```python
from build123d import *

# Parameters (mm, degrees)
SM_BASE_FLANGE_1_DEPTH = 80
CUT_EXTRUDE_1_DEPTH    = 35
FILLET_1_R             = 1
EXTRUDE_START          = -1.5
EXTRUDE_1_OUTLINE_R    = 4.25
EXTRUDE_1_DEPTH        = 1.5


# Read off the part's stored shape, not the designer's step: Бобышка-Вытянуть1
# Sheet-metal steps are written as plain solids
with BuildPart() as part:
    # Sketch 1 → Базовая кромка1 (new body)
    with BuildSketch(Plane(origin=(0, 0, 0), x_dir=(0, 0, -1), z_dir=(1, 0, 0))):
        with BuildLine():
            Line((-6, 25.5), (-6, 1))
            ThreePointArc((-6, 1), (-5.707106781, 0.292893219), (-5, 0))
            Line((-5, 0), (5, 0))
            ThreePointArc((5, 0), (5.707106781, 0.292893219), (6, 1))
            Line((6, 1), (6, 25.5))
            Line((6, 25.5), (7.5, 25.5))
            Line((7.5, 25.5), (7.5, 1))
            ThreePointArc((7.5, 1), (6.767766953, -0.767766953), (5, -1.5))
            Line((5, -1.5), (-5, -1.5))
            ThreePointArc((-5, -1.5), (-6.767766953, -0.767766953), (-7.5, 1))
            Line((-7.5, 1), (-7.5, 25.5))
            Line((-7.5, 25.5), (-6, 25.5))
        make_face()
    extrude(amount=SM_BASE_FLANGE_1_DEPTH)

    # Эскиз6 → Вырез-Вытянуть1 (cut)
    with BuildSketch(Plane.XY.offset(7.5)):
        Polygon((80, 25.5), (75.076809621, 25.5), (80, 5.5), align=None)
        with BuildLine():
            ThreePointArc((13.923190379, 25.5), (23.568323275, 11.075714714), (40, 5.5))
            Line((40, 5.5), (40, 25.5))
            Line((40, 25.5), (13.923190379, 25.5))
        make_face()
        with BuildLine():
            Line((40, 25.5), (40, 5.5))
            ThreePointArc((40, 5.5), (56.431676725, 11.075714714), (66.076809621, 25.5))
            Line((66.076809621, 25.5), (40, 25.5))
        make_face()
        Polygon((0, 5.5), (4.923190379, 25.5), (0, 25.5), align=None)
    extrude(amount=-CUT_EXTRUDE_1_DEPTH, mode=Mode.SUBTRACT)

    # Скругление1
    fillet_1_edges = [part.edges().sort_by_distance(p)[0] for p in [
        (75.076809621, 25.5, -6.75),
        (75.076809621, 25.5, 6.75),
        (13.923190379, 25.5, -6.75),
        (66.076809621, 25.5, -6.75),
        (13.923190379, 25.5, 6.75),
        (66.076809621, 25.5, 6.75),
        (4.923190379, 25.5, -6.75),
        (4.923190379, 25.5, 6.75),
    ]]
    fillet(fillet_1_edges, radius=FILLET_1_R)

    # Бобышка-Вытянуть1 outline → Бобышка-Вытянуть1 (cut)
    with BuildSketch(Plane.XZ.offset(1.5).offset(EXTRUDE_START)):
        with Locations((71, 0)):
            Circle(EXTRUDE_1_OUTLINE_R)
        with Locations((9, 0)):
            Circle(EXTRUDE_1_OUTLINE_R)
    extrude(amount=EXTRUDE_1_DEPTH, mode=Mode.SUBTRACT)


solid = part.part
```
Work out the finished part from the listing and answer in its coordinate system (mm). A direction names the side the tool comes from. Give positions to 0.01 mm unless a question says otherwise; leave off trailing zeros. Loops run counter-clockwise (first coordinate to the right, second up) from the corner with the lowest first, then second, coordinate; pieces in that order, holes last. Notation, with made-up numbers: (16.25, 27.25) -> (59.25, 27.25) arc R3 ccw to (59.25, 32.25) -> close; hole circle Ø10 at (3.25, 39). An arc over 180 degrees is marked (long way). Write item = value, one per line. Start each with the question number.
(1) Find the intervals of material crossed by probe 1 along Z at (x, y) = (71.5, 15); probe 2 along Y at (x, z) = (73, 4.75); probe 3 along Z at (x, y) = (9, -0.8), in increasing order. Write a range as from..to.
(2) Find section C-C on z = 0. Give the vertices of the cut face in (x, y).
(3) Find section A-A on x = 71. Give the vertices of the cut face in (y, z), and give its area (3 significant figures).
(4) Which of the six approach directions +Z, -Z, +X, -X, +Y, -Y give full straight-line access (tool end or side, diameter ignored) to faces 4 (the flat face through (39, 5, -6)), 5 (the cylindrical face through (39.44, -0.748, -6.787))?
(5) Given pin 1 Ø5 at (y, z) = (15, -4) entering from -X; pin 2 Ø1.5 at (x, z) = (55.5, -1) entering from +Y; pin 3 Ø6 at (y, z) = (13, -5) entering from +X; pin 4 Ø12 at (x, y) = (49, 20.5) entering from -Z, each flat-ended and moving along its own axis, determine where each tip first touches the part or whether it passes through.
(6) Find section D-D on x = 41. Give the vertices of the cut face in (y, z).
(7) The mould has two halves that part along Z. Classify faces 1 (the flat face through (39, 5, 6)), 2 (the cylindrical face through (39.44, -0.787, 6.748)), 3 (the flat face through (2.335, 14.985, -6.74)): +Z half, -Z half, draft (parallel to the pull), parting line (faces both ways), or undercut.
(8) Find section B-B on y = 16.75. Give the vertices of the cut face in (x, z), and give its area (3 significant figures).
From the geometry:
q1.probe_1 = -7.5..-6, 6..7.5
q1.probe_2 = -1.5..0
q1.probe_3 = -6.73..-4.25, 4.25..6.73
q2.outline = (0, -1.5) -> (4.75, -1.5) -> (4.75, 0) -> (0, 0) -> close; (13.25, -1.5) -> (66.75, -1.5) -> (66.75, 0) -> (13.25, 0) -> close; (75.25, -1.5) -> (80, -1.5) -> (80, 0) -> (75.25, 0) -> close
q3.outline = (-1.5, -5) arc R2.5 ccw to (1, -7.5) -> (25.5, -7.5) -> (25.5, -6) -> (1, -6) arc R1 cw to (0, -5) -> (0, -4.25) -> (-1.5, -4.25) -> close; (-1.5, 4.25) -> (0, 4.25) -> (0, 5) arc R1 cw to (1, 6) -> (25.5, 6) -> (25.5, 7.5) -> (1, 7.5) arc R2.5 ccw to (-1.5, 5) -> close
q3.area = 84.0 mm^2
q4.face_4 = +X, -X, +Y
q4.face_5 = -Z, +X, -X, -Y
q5.pin_1 = 1.97
q5.pin_2 = 0
q5.pin_3 = 78.85
q5.pin_4 = through
q6.outline = (-1.5, -5) arc R2.5 ccw to (1, -7.5) -> (5.52, -7.5) -> (5.52, -6) -> (1, -6) arc R1 cw to (0, -5) -> (0, 5) arc R1 cw to (1, 6) -> (5.52, 6) -> (5.52, 7.5) -> (1, 7.5) arc R2.5 ccw to (-1.5, 5) -> close
q7.face_1 = undercut
q7.face_2 = +Z half
q7.face_3 = draft
q8.outline = (2.77, -7.5) -> (18.07, -7.5) -> (18.07, -6) -> (2.77, -6) -> close; (2.77, 6) -> (18.07, 6) -> (18.07, 7.5) -> (2.77, 7.5) -> close; (61.93, -7.5) -> (77.23, -7.5) -> (77.23, -6) -> (61.93, -6) -> close; (61.93, 6) -> (77.23, 6) -> (77.23, 7.5) -> (61.93, 7.5) -> close
q8.area = 91.8 mm^2
